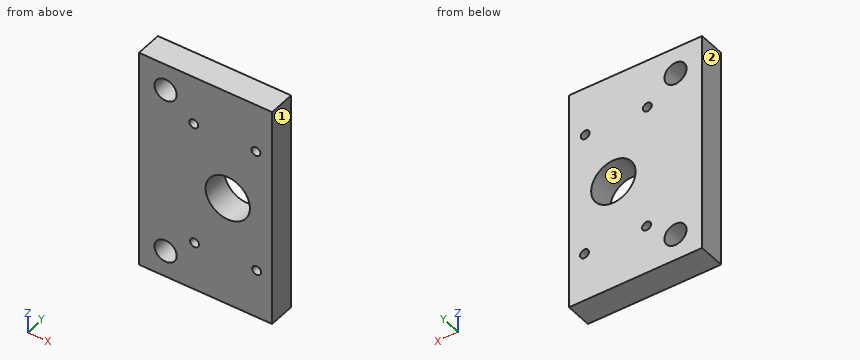
```python
from build123d import *

# Parameters (mm, degrees)
F0_R     = 12.5
F0_R_2   = 5
F0_R_3   = 25
F1_DEPTH = 30


with BuildPart() as f1:
    # F0 (on Front) → F1 (new body)
    with BuildSketch(Plane.XZ):
        Polygon((75, -70), (75, 125), (-75, 125), (-75, -125), (75, -125), align=None)
        with Locations((-45, -95)):
            Circle(F0_R, mode=Mode.SUBTRACT)
        with Locations((-12.458926, -70)):
            Circle(F0_R_2, mode=Mode.SUBTRACT)
        with Locations((57.541074, -70)):
            Circle(F0_R_2, mode=Mode.SUBTRACT)
        with Locations((-45, 95)):
            Circle(F0_R, mode=Mode.SUBTRACT)
        with Locations((-13.282487, 70)):
            Circle(F0_R_2, mode=Mode.SUBTRACT)
        with Locations((25, 0)):
            Circle(F0_R_3, mode=Mode.SUBTRACT)
        with Locations((56.717513, 70)):
            Circle(F0_R_2, mode=Mode.SUBTRACT)
    extrude(amount=F1_DEPTH)


solid = f1.part
```
Work out the finished part from the listing and answer in its coordinate system (mm). Face numbers are marked on the shaded views. Give positions to 0.01 mm unless a question says otherwise; leave off trailing zeros. Loops run counter-clockwise (first coordinate to the right, second up) from the corner with the lowest first, then second, coordinate; pieces in that order, holes last. Notation, with made-up numbers: (85.25, 60.25) - (102.25, 60.25) arc R20 cw to (102.25, 68.25) - close; hole circle Ø9 at (41, 75.5). An arc over 180 degrees is marked (long way). One line per question, with ' | ' between items.
(1) The part is cut by section D-D (z = -70). Write down the section's boundary in (x, y).
Recorded:
outline: (-75, -30) - (-17.46, -30) - (-17.46, 0) - (-75, 0) - close; (-7.46, -30) - (52.54, -30) - (52.54, 0) - (-7.46, 0) - close; (62.54, -30) - (75, -30) - (75, 0) - (62.54, 0) - close
(2) The part is cut by section C-C (x = 25). Write down the section's boundary in (y, z), then the cut area to 3 significant figures.
Recorded:
outline: (-30, -125) - (0, -125) - (0, -25) - (-30, -25) - close; (-30, 25) - (0, 25) - (0, 125) - (-30, 125) - close | area: 6,000 mm²
(3) Straight lines are drawn through the part: probe 1 along X at (y, z) = (-10, 1.5); probe 2 along Z at (x, y) = (25, -19); probe 3 along Z at (x, y) = (-16.5, -15). For each, find the intervals that lie inside material, in ascending order.
Recorded:
probe 1: x = -75 to 0.05, 49.95 to 75 | probe 2: z = -125 to -25, 25 to 125 | probe 3: z = -125 to -72.94, -67.06 to 66.17, 73.83 to 125
(4) The part is cut by section A-A (x = -45). Write down the section's boundary in (y, z).
Recorded:
outline: (-30, -125) - (0, -125) - (0, -107.5) - (-30, -107.5) - close; (-30, -82.5) - (0, -82.5) - (0, 82.5) - (-30, 82.5) - close; (-30, 107.5) - (0, 107.5) - (0, 125) - (-30, 125) - close
(5) The mould has two halves that part along X. Classify the marked faces 1, 2 and 3: +X half, -X half, draft (parallel to the pull), parting line (faces both ways), or undercut.
Recorded:
face 1: +X half | face 2: -X half | face 3: undercut
(6) The part is cut by section B-B (z = 95). Write down the section's boundary in (x, y).
Recorded:
outline: (-75, -30) - (-57.5, -30) - (-57.5, 0) - (-75, 0) - close; (-32.5, -30) - (75, -30) - (75, 0) - (-32.5, 0) - close
(7) This flat-tipped pin is pushed along its axis until it touches: pin 1 Ø9 at (x, z) = (-12.46, -70) entering from -Y. Where does it stop, or does it pass through?
Recorded:
pin 1: passes through
